Solid Edge part; units mm, degrees
sketch "Sketch1" plane through (0, 0, 0) normal (0, 0, 1) x (1, 0, 0)
  line L0 (5.35, 8.4485) -> (5.35, -8.4485)
  arc A0 (5.35, -8.4485) -> (5.35, 8.4485) centre (0, 0) cw
  line L1 (-2.35, -2.9223) -> (-2.35, 2.9223)
  arc A1 (2.35, -2.9223) -> (-2.35, -2.9223) centre (0, 0) cw
  line L2 (2.35, 2.9223) -> (2.35, -2.9223)
  arc A2 (-2.35, 2.9223) -> (2.35, 2.9223) centre (0, 0) cw
extrude "Protrusion1" add sketch "Sketch1" along normal blind 10
fillet "Round_1" radius 2 1 edges at (5.35, 8.4485, 5)
fillet "Round_2" radius 2 1 edges at (5.35, -8.4485, 5)
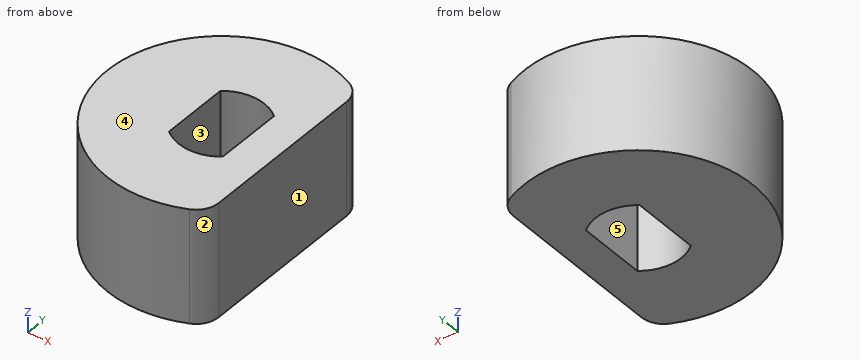
Verification items for the finished model (mm, model axes). Face numbers are marked on the shaded views. A direction names the side the tool comes from. Round coordinates to 2 decimals unless told otherwise and drop trailing zeros. Write each loop counter-clockwise with the first axis right and the second up, starting at its lowest first coordinate (ties: lowest second). Pieces come first, ordered by that corner, then holes. Notation, with made-up numbers: (73.25, -26.75) - (92.25, -26.75) arc R15 ccw to (92.25, -7.75) - close; hole circle Ø8 at (-0.5, 5). An arc over 180 degrees is marked (long way). Answer as a JSON object with one key per item and string values. Group by question number.
Q1. Thickness scan on line 1 (Y direction, x = -2, z = 1.25); line 2 (X direction, y = -1.5, z = 2.25); line 3 (X direction, y = 2.25, z = 1). Record the ranges inside material, lowest first.
Q2. Mould release check, pull along Y, two halves, no side actions. Record for the marked faces 1, 2 and 3: released by +Y, released by -Y, zero draft, split by the parting line, or undercut.
Q3. Section check A-A, the plane y = 0. Enter the section's corners in (x, z).
Q4. Section check D-D, the plane y = 6.5. Enter the section's corners in (x, z).
Q5. Tool access check on the marked faces 4 and 5. Record the directions out of +Z, -Z, +X, -X, +Y, -Y that give a thin tool (end or side, any length) a straight path to the whole face; none if there is none.
Q6. Section check C-C, the plane z = 8. Enter the section's corners in (x, y), plus the area to 3 significant figures.
Q7. Section check B-B, the plane x = 0. Enter the section's corners in (y, z), plus the area to 3 significant figures.
Q8. Go/stop test with flat-tipped pins: pin 1 Ø5 at (x, z) = (-2, 4.5) entering from +Y; pin 2 Ø1.5 at (x, z) = (3.5, 4.5) entering from -Y. Record where each tip stops, or that it passes through.
Found:
{
 "1": {"line 1": "y = -9.8 to -3.17, 3.17 to 9.8", "line 2": "x = -9.89 to -2.35, 2.35 to 5.35", "line 3": "x = -9.74 to -2.35, 2.35 to 5.35"},
 "2": {"face 1": "zero draft", "face 2": "released by -Y", "face 3": "undercut"},
 "3": {"outline": "(-10, 0) - (-2.35, 0) - (-2.35, 10) - (-10, 10) - close; (2.35, 0) - (5.35, 0) - (5.35, 10) - (2.35, 10) - close"},
 "4": {"outline": "(-7.6, 0) - (5.35, 0) - (5.35, 10) - (-7.6, 10) - close"},
 "5": {"face 4": "+Z, +X, -X, +Y, -Y", "face 5": "+Z, -Z"},
 "6": {"outline": "(4.19, -9.08) arc R2 ccw to (5.35, -7.26) - (5.35, 7.26) arc R2 ccw to (4.19, 9.08) arc R10 ccw (long way) to start; hole (-2.35, -2.92) arc R3.75 ccw to (2.35, -2.92) - (2.35, 2.92) arc R3.75 ccw to (-2.35, 2.92) - close", "area": "225 mm^2"},
 "7": {"outline": "(-10, 0) - (-3.75, 0) - (-3.75, 10) - (-10, 10) - close; (3.75, 0) - (10, 0) - (10, 10) - (3.75, 10) - close", "area": "125 mm^2"},
 "8": {"pin 1": "stops at y = 10", "pin 2": "stops at y = -9.61"}
}
